```python
from build123d import *

# Parameters (mm, degrees)
F1_DEPTH  = 44.45
F9_DEPTH  = 9.525
F10_DEPTH = 9.525
F12_DEPTH = 2.38125
F13_R     = 11.7475
F13_R_2   = 10.7315
F14_DEPTH = 7.9375
F15_DEPTH = 10.31875
F16_W     = 26.9525004551
F16_H     = 57.8892836347
F17_DEPTH = 12.7
F19_W     = 21.59
F19_H     = 54.76875
F20_DEPTH = 2.54
F27_DEPTH = 25.4


with BuildPart() as f1:
    # F0 (on Top) → F1 (new body)
    with BuildSketch(Plane.XY):
        with BuildLine():
            ThreePointArc((-4.572, 0), (0, 4.572), (4.572, 0))
            Line((4.572, 0), (7.747, 0))
            ThreePointArc((7.747, 0), (5.951410253, 4.9595085442), (1.397, 7.62))
            ThreePointArc((1.397, 7.62), (0, 7.747), (-1.397, 7.62))
            ThreePointArc((-1.397, 7.62), (-5.951410253, 4.9595085442), (-7.747, 0))
            Line((-7.747, 0), (-4.572, 0))
        make_face()
        with BuildLine():
            ThreePointArc((-1.397, 7.62), (0, 7.747), (1.397, 7.62))
            Line((1.397, 7.62), (1.397, 19.3802))
            ThreePointArc((1.397, 19.3802), (0, 19.1615406713), (-1.397, 19.3802))
            Line((-1.397, 19.3802), (-1.397, 7.62))
        make_face()
        with BuildLine():
            ThreePointArc((-1.397, 19.3802), (0, 19.1615406713), (1.397, 19.3802))
            ThreePointArc((1.397, 19.3802), (3.6939320514, 21.0394638349), (4.572, 23.7335406713))
            ThreePointArc((4.572, 23.7335406713), (-2.6940768363, 27.4274727226), (-1.397, 19.3802))
        make_face()
    extrude(amount=F1_DEPTH)

    # F6 (on offset) → F9 (cut)
    with BuildSketch(Plane.XY.offset(28.575)):
        with BuildLine():
            ThreePointArc((4.1557772601, 1.7640375299), (0, -1.016), (-4.1557772601, 1.7640375299))
            Line((-4.1557772601, 1.7640375299), (-7.6070004234, 1.7640375299))
            ThreePointArc((-7.6070004234, 1.7640375299), (0, -4.318), (7.6070004234, 1.7640375299))
            Line((7.6070004234, 1.7640375299), (4.1557772601, 1.7640375299))
        make_face()
        with BuildLine():
            ThreePointArc((-4.1557772601, 1.7640375299), (-0.8747878771, 7.8904367738), (4.4961791045, 3.4801791045))
            ThreePointArc((4.4961791045, 3.4801791045), (4.4102576693, 2.6053912274), (4.1557772601, 1.7640375299))
            Line((4.1557772601, 1.7640375299), (7.6070004234, 1.7640375299))
            ThreePointArc((7.6070004234, 1.7640375299), (7.750237064, 2.6168003938), (7.7981791045, 3.4801791045))
            ThreePointArc((7.7981791045, 3.4801791045), (-0.8633787106, 11.2304161684), (-7.6070004234, 1.7640375299))
            Line((-7.6070004234, 1.7640375299), (-4.1557772601, 1.7640375299))
        make_face()
        with BuildLine():
            ThreePointArc((7.6070004234, 1.7640375299), (0, -4.318), (-7.6070004234, 1.7640375299))
            Line((-7.6070004234, 1.7640375299), (-8.4216929972, 1.7640375299))
            Line((-8.4216929972, 1.7640375299), (-8.4216929972, -6.3198274001))
            Line((-8.4216929972, -6.3198274001), (11.7628639564, -6.3198274001))
            Line((11.7628639564, -6.3198274001), (11.7628639564, 1.7640375299))
            Line((11.7628639564, 1.7640375299), (7.6070004234, 1.7640375299))
        make_face()
    extrude(amount=F9_DEPTH, mode=Mode.SUBTRACT)

    # F8 (on offset) → F10 (cut)
    with BuildSketch(Plane.XY.offset(15.875)):
        with BuildLine():
            ThreePointArc((4.179462045, 1.8225532258), (0, -1.016), (-4.179462045, 1.8225532258))
            Line((-4.179462045, 1.8225532258), (-7.6199654718, 1.8225532258))
            ThreePointArc((-7.6199654718, 1.8225532258), (0, -4.318), (7.6199654718, 1.8225532258))
            Line((7.6199654718, 1.8225532258), (4.179462045, 1.8225532258))
        make_face()
        with BuildLine():
            ThreePointArc((-4.179462045, 1.8225532258), (-0.8438058499, 7.8964692022), (4.4961791045, 3.4801791045))
            ThreePointArc((4.4961791045, 3.4801791045), (4.4162900977, 2.6363732546), (4.179462045, 1.8225532258))
            Line((4.179462045, 1.8225532258), (7.6199654718, 1.8225532258))
            ThreePointArc((7.6199654718, 1.8225532258), (7.7534976902, 2.6465899292), (7.7981791045, 3.4801791045))
            ThreePointArc((7.7981791045, 3.4801791045), (-0.8335891753, 11.2336767947), (-7.6199654718, 1.8225532258))
            Line((-7.6199654718, 1.8225532258), (-4.179462045, 1.8225532258))
        make_face()
        with BuildLine():
            ThreePointArc((7.6199654718, 1.8225532258), (0, -4.318), (-7.6199654718, 1.8225532258))
            Line((-7.6199654718, 1.8225532258), (-8.5849482566, 1.8225532258))
            Line((-8.5849482566, 1.8225532258), (-8.5849482566, -5.9901881032))
            Line((-8.5849482566, -5.9901881032), (8.4006469697, -5.9901881032))
            Line((8.4006469697, -5.9901881032), (8.4006469697, 1.8225532258))
            Line((8.4006469697, 1.8225532258), (7.6199654718, 1.8225532258))
        make_face()
    extrude(amount=-F10_DEPTH, mode=Mode.SUBTRACT)

    # F11 (on face) → F12 (join)
    with BuildSketch(Plane.XY.offset(44.45)):
        with BuildLine():
            ThreePointArc((-1.397, 11.6641393703), (-7.7971949684, -8.7867802337), (11.7475, 0))
            ThreePointArc((11.7475, 0), (8.7867802337, 7.7971949684), (1.397, 11.6641393703))
            Line((1.397, 11.6641393703), (1.397, 7.62))
            ThreePointArc((1.397, 7.62), (5.951410253, 4.9595085442), (7.747, 0))
            Line((7.747, 0), (4.572, 0))
            ThreePointArc((4.572, 0), (0, -4.572), (-4.572, 0))
            Line((-4.572, 0), (-7.747, 0))
            ThreePointArc((-7.747, 0), (-5.951410253, 4.9595085442), (-1.397, 7.62))
            Line((-1.397, 7.62), (-1.397, 11.6641393703))
        make_face()
        with BuildLine():
            Line((1.397, 7.62), (1.397, 11.6641393703))
            ThreePointArc((1.397, 11.6641393703), (0, 11.7475), (-1.397, 11.6641393703))
            Line((-1.397, 11.6641393703), (-1.397, 7.62))
            ThreePointArc((-1.397, 7.62), (-5.951410253, 4.9595085442), (-7.747, 0))
            Line((-7.747, 0), (-4.572, 0))
            ThreePointArc((-4.572, 0), (0, 4.572), (4.572, 0))
            Line((4.572, 0), (7.747, 0))
            ThreePointArc((7.747, 0), (5.951410253, 4.9595085442), (1.397, 7.62))
        make_face()
    extrude(amount=F12_DEPTH)

    # F13 (on face) → F14 (join)
    with BuildSketch(Plane.XY.offset(46.83125)):
        Circle(F13_R)
        Circle(F13_R_2, mode=Mode.SUBTRACT)
    extrude(amount=F14_DEPTH)

    # F15 (add, through all): a face of the model
    f15_faces = [f1.faces().sort_by_distance(p)[0] for p in [
        (0, 21.7334038121, 44.45),
    ]]
    extrude(f15_faces, amount=F15_DEPTH)

    # F16 (on Right) → F17 (cut, symmetric)
    with BuildSketch(Plane.YZ):
        with Locations((26.0822460987, 27.6629510336)):
            Rectangle(F16_W, F16_H)
    extrude(amount=F17_DEPTH, both=True, mode=Mode.SUBTRACT)



with BuildPart() as f20:
    # F19 (on offset) → F20 (new body)
    with BuildSketch(Plane(origin=(0, 12.6059958711, 0), x_dir=(-1, 0, 0), z_dir=(0, 1, 0))):
        with Locations((0, 27.384375)):
            Rectangle(F19_W, F19_H)
    extrude(amount=F20_DEPTH)

    # F24: sweep along a path in F23
    with BuildLine(Plane(origin=(0, 15.1459958711, 0), x_dir=(-1, 0, 0), z_dir=(0, 1, 0))) as f24_path:
        Line((0, 27.384375), (5.8207285935, 54.76875))
    # F22 (on mid) → F24 (sweep)
    with BuildSketch(Plane.XY.offset(27.384375)):
        with BuildLine():
            ThreePointArc((4.572, 27.3733365424), (-2.6940768363, 31.0672685937), (-1.397, 23.0199958711))
            ThreePointArc((-1.397, 23.0199958711), (0, 22.8013365424), (1.397, 23.0199958711))
            ThreePointArc((1.397, 23.0199958711), (3.6939320514, 24.6792597061), (4.572, 27.3733365424))
        make_face()
        with BuildLine():
            Line((-1.397, 23.0199958711), (-1.397, 15.1459958711))
            Line((-1.397, 15.1459958711), (1.397, 15.1459958711))
            Line((1.397, 15.1459958711), (1.397, 23.0199958711))
            ThreePointArc((1.397, 23.0199958711), (0, 22.8013365424), (-1.397, 23.0199958711))
        make_face()
    sweep(path=f24_path.line)


with BuildPart() as f1_1:
    add(f1.part)

    add(f20.part)  # F25 merges F20
    # F25: sweep along a path in F23
    with BuildLine(Plane(origin=(0, 15.1459958711, 0), x_dir=(-1, 0, 0), z_dir=(0, 1, 0))) as f25_path:
        Line((-5.8207285935, 0), (0, 27.384375))
    # F22 (on mid) → F25 (sweep)
    with BuildSketch(Plane.XY.offset(27.384375)):
        with BuildLine():
            Line((-1.397, 23.0199958711), (-1.397, 15.1459958711))
            Line((-1.397, 15.1459958711), (1.397, 15.1459958711))
            Line((1.397, 15.1459958711), (1.397, 23.0199958711))
            ThreePointArc((1.397, 23.0199958711), (0, 22.8013365424), (-1.397, 23.0199958711))
        make_face()
        with BuildLine():
            ThreePointArc((4.572, 27.3733365424), (-2.6940768363, 31.0672685937), (-1.397, 23.0199958711))
            ThreePointArc((-1.397, 23.0199958711), (0, 22.8013365424), (1.397, 23.0199958711))
            ThreePointArc((1.397, 23.0199958711), (3.6939320514, 24.6792597061), (4.572, 27.3733365424))
        make_face()
    sweep(path=f25_path.line)

    # F26 (on face) → F27 (cut)
    with BuildSketch(Plane.XZ.offset(-12.6059958711)):
        Polygon((7.747, 0), (3.5317886158, -0.8959708385), (7.8619366049, -6.503867323), (24.6146406516, -1.8187895067), (20.6104957086, 2.7342204189), (10.795, 0.6478724), (10.795, 0), align=None)
        Polygon((10.795, 0.6478724), (7.747, 0), (10.795, 0), align=None)
    extrude(amount=-F27_DEPTH, mode=Mode.SUBTRACT)


solid = f1_1.part
```
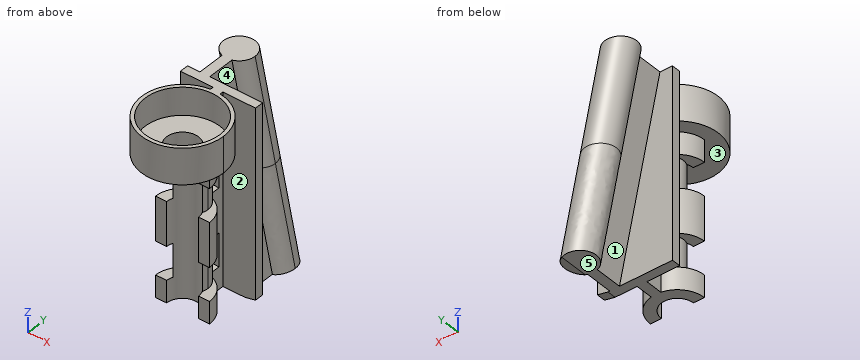
For this review, take the finished solid that the model builds, in its own axes (mm). Face numbers are marked on the shaded views. A direction names the side the tool comes from. Round coordinates to 2 decimals unless told otherwise and drop trailing zeros. Write each loop counter-clockwise with the first axis right and the second up, starting at its lowest first coordinate (ties: lowest second). Pieces come first, ordered by that corner, then holes. Notation, with made-up numbers: (12.25, 24.25) -> (17.25, 24.25) arc R23 ccw to (17.25, 53.25) -> close; hole circle Ø10 at (-9.5, 7.5). An arc over 180 degrees is marked (long way). One line per question, with ' | ' between items. Start each with the question number.
1) Machinability: for the marked faces 1, 2 and 3, which of the approach directions +Z, -Z, +X, -X, +Y, -Y give a long, thin tool a straight path to every point of the face, cutting with its end or side? Answer none if there is none.
2) Add section B-B (x = 0). Count the separate pieces of the cut face and the enclosed holes in it, and give its area (3 significant figures).
3) Mouldability with a two-part tool opening along Y and no side actions: class the marked faces 4 and 5 as +Y half, -Y half, draft (parallel to the pull), parting line (faces both ways), or undercut.
4) For pin 1 Ø1.5 at (x, z) = (-6.5, 29) entering from -Y; pin 2 Ø5.5 at (y, z) = (11, 20) entering from -X (3 decimals); pin 3 Ø1 at (x, z) = (-7, 33.5) entering from +Y, all flat-tipped, find the tip position at first contact; note any pin that passes through.
5) Wall thickness on line 1 along Y through (x, z) = (-7, 47.5); line 2 along Y through (x, z) = (0, 51.75); line 3 along Y through (x, z) = (0, 26): over which ranges is each line inside the solid? List them lowest first.
6) Add section A-A (y = -3.5). Write out the cut boundary in (x, z), and give its area (3 significant figures).
Reported:
1) face 1: -Z, -X | face 2: +Z, -Z, +X | face 3: -Z
2) separate pieces: 2 | enclosed holes: 2 | area: 903 mm²
3) face 4: undercut | face 5: draft
4) pin 1: stops at y = 0 | pin 2: stops at x = -10.795 | pin 3: stops at y = 15.15
5) line 1: y = -9.43 to -8.13, 8.13 to 9.43, 12.61 to 15.15, 23.7 to 31.05 | line 2: y = -11.75 to -10.73, 10.73 to 15.15 | line 3: y = 4.57 to 31.94
6) outline: (-11.21, 44.45) -> (-2.94, 44.45) -> (-2.94, 46.83) -> (-10.14, 46.83) -> (-10.14, 54.77) -> (-11.21, 54.77) -> close; (2.94, 44.45) -> (11.21, 44.45) -> (11.21, 54.77) -> (10.14, 54.77) -> (10.14, 46.83) -> (2.94, 46.83) -> close | area: 56.4 mm²
